The listing builds one solid part. Answer for the finished solid, in the listing's coordinates (mm). Coordinates: 2 decimals unless noted, no trailing zeros. Loops run counter-clockwise (first coordinate to the right, second up) from the corner with the lowest first, then second, coordinate; pieces in that order, holes last. Notation, with made-up numbers: (68, 28.25) - (94, 28.25) arc R29 cw to (94, 51.25) - close; hole circle Ø3 at (49, -26.5). An arc over 180 degrees is marked (long way). Return JSON: item names as keys, results as strings. Group by question number.
1. Section A-A (z = 0) is taken. Write down the section's boundary in (x, y).
2. Section D-D (y = 3.35) is taken. State how many separate pieces and enclosed holes the cut face has, and give its area (3 significant figures).
3. Each of these flat-tipped pins is pushed along its axis until it touches: P1, Ø2.5, axis at x = -40.66, z = 32.42, coming from the -Y side; P2, Ø1, axis at x = -24.5, y = 2.5, coming from the +Z side; P3, Ø1, axis at x = 4, y = 3, coming from the -Z side. Where does it stop, or does it pass through?
4. The mould has two halves that part along X. Classify faces 1 (the face through (-42.98, 2.03, -17.76)), 2 (the face through (13.836, 1.972, -23.766)): pulls with the +X half, pulls with the -X half, needs draft (parallel to the pull), parting line crosses it, or undercut.
5. Find the intervals of material crossed by line 1 along X through (y, z) = (3, -5); line 2 along X through (y, z) = (3.8, -22); line 3 along Z through (x, y) = (21, 1.3), in increasing order.
6. Section C-C (z = -36) is taken. Write down the section's boundary in (x, y).
7. Section B-B (x = 0) is taken. Write down the section's boundary in (y, z), and give its area (3 significant figures).
```python
from build123d import *

# Parameters (mm, degrees)
SKETCH_1_R      = 56
SKETCH_1_R_2    = 2.6
SKETCH_1_R_3    = 17.5
SKETCH_1_R_4    = 1.5
EXTRUDE_1_DEPTH = 4
FILLET_1_R      = 3


with BuildPart() as part:
    # 草图1 → 凸台-拉伸1 (new body)
    with BuildSketch(Plane(origin=(0, 0, 0), x_dir=(1, 0, 0), z_dir=(0, 1, 0))):
        with Locations(Location((0, 0, 0), (0, 0, 270))):
            Circle(SKETCH_1_R)
        with BuildLine():
            Line((-5, 47.236109069), (-5, 27.041634566))
            ThreePointArc((-5, 27.041634566), (-13.75, 23.815698604), (-20.918742494, 17.850944302))
            Line((-20.918742494, 17.850944302), (-38.40767043, 27.948181554))
            ThreePointArc((-38.40767043, 27.948181554), (-23.75, 41.13620668), (-5, 47.236109069))
        make_face(mode=Mode.SUBTRACT)
        with BuildLine():
            Line((-43.40767043, 19.287927516), (-25.918742494, 9.190690264))
            ThreePointArc((-25.918742494, 9.190690264), (-27.5, 0), (-25.918742494, -9.190690264))
            Line((-25.918742494, -9.190690264), (-43.40767043, -19.287927516))
            ThreePointArc((-43.40767043, -19.287927516), (-47.5, 0), (-43.40767043, 19.287927516))
        make_face(mode=Mode.SUBTRACT)
        with BuildLine():
            Line((-38.40767043, -27.948181554), (-20.918742494, -17.850944302))
            ThreePointArc((-20.918742494, -17.850944302), (-13.75, -23.815698604), (-5, -27.041634566))
            Line((-5, -27.041634566), (-5, -47.236109069))
            ThreePointArc((-5, -47.236109069), (-23.75, -41.13620668), (-38.40767043, -27.948181554))
        make_face(mode=Mode.SUBTRACT)
        with BuildLine():
            Line((5, -47.236109069), (5, -27.041634566))
            ThreePointArc((5, -27.041634566), (13.75, -23.815698604), (20.918742494, -17.850944302))
            Line((20.918742494, -17.850944302), (38.40767043, -27.948181554))
            ThreePointArc((38.40767043, -27.948181554), (23.75, -41.13620668), (5, -47.236109069))
        make_face(mode=Mode.SUBTRACT)
        with BuildLine():
            Line((43.40767043, -19.287927516), (25.918742494, -9.190690264))
            ThreePointArc((25.918742494, -9.190690264), (27.5, 0), (25.918742494, 9.190690264))
            Line((25.918742494, 9.190690264), (43.40767043, 19.287927516))
            ThreePointArc((43.40767043, 19.287927516), (47.5, 0), (43.40767043, -19.287927516))
        make_face(mode=Mode.SUBTRACT)
        with BuildLine():
            Line((38.40767043, 27.948181554), (20.918742494, 17.850944302))
            ThreePointArc((20.918742494, 17.850944302), (13.75, 23.815698604), (5, 27.041634566))
            Line((5, 27.041634566), (5, 47.236109069))
            ThreePointArc((5, 47.236109069), (23.75, 41.13620668), (38.40767043, 27.948181554))
        make_face(mode=Mode.SUBTRACT)
        with Locations(Location((0, 22.5, 0), (0, 0, 270))):
            Circle(SKETCH_1_R_2, mode=Mode.SUBTRACT)
        with Locations(Location((-19.485571585, -11.25, 0), (0, 0, 270))):
            Circle(SKETCH_1_R_2, mode=Mode.SUBTRACT)
        with Locations(Location((0, -22.5, 0), (0, 0, 270))):
            Circle(SKETCH_1_R_2, mode=Mode.SUBTRACT)
        with Locations(Location((19.485571585, -11.25, 0), (0, 0, 270))):
            Circle(SKETCH_1_R_2, mode=Mode.SUBTRACT)
        with Locations(Location((-19.485571585, 11.25, 0), (0, 0, 270))):
            Circle(SKETCH_1_R_2, mode=Mode.SUBTRACT)
        with Locations(Location((0, 0, 0), (0, 0, 270))):
            Circle(SKETCH_1_R_3, mode=Mode.SUBTRACT)
        with Locations(Location((19.485571585, 11.25, 0), (0, 0, 270))):
            Circle(SKETCH_1_R_2, mode=Mode.SUBTRACT)
        with Locations(Location((-32.421469697, -40.655237088, 0), (0, 0, 270))):
            Circle(SKETCH_1_R_4, mode=Mode.SUBTRACT)
        with Locations(Location((-40.655237088, -32.421469697, 0), (0, 0, 270))):
            Circle(SKETCH_1_R_4, mode=Mode.SUBTRACT)
        with Locations(Location((-22.561954434, -46.850381131, 0), (0, 0, 270))):
            Circle(SKETCH_1_R_4, mode=Mode.SUBTRACT)
        with Locations(Location((-11.571088566, -50.696251433, 0), (0, 0, 270))):
            Circle(SKETCH_1_R_4, mode=Mode.SUBTRACT)
        with Locations(Location((-46.850381131, -22.561954434, 0), (0, 0, 270))):
            Circle(SKETCH_1_R_4, mode=Mode.SUBTRACT)
        with Locations(Location((-50.696251433, -11.571088566, 0), (0, 0, 270))):
            Circle(SKETCH_1_R_4, mode=Mode.SUBTRACT)
        with Locations(Location((-52, 0, 0), (0, 0, 270))):
            Circle(SKETCH_1_R_4, mode=Mode.SUBTRACT)
        with Locations(Location((0, -52, 0), (0, 0, 270))):
            Circle(SKETCH_1_R_4, mode=Mode.SUBTRACT)
        with Locations(Location((11.571088566, -50.696251433, 0), (0, 0, 270))):
            Circle(SKETCH_1_R_4, mode=Mode.SUBTRACT)
        with Locations(Location((22.561954434, -46.850381131, 0), (0, 0, 270))):
            Circle(SKETCH_1_R_4, mode=Mode.SUBTRACT)
        with Locations(Location((32.421469697, -40.655237088, 0), (0, 0, 270))):
            Circle(SKETCH_1_R_4, mode=Mode.SUBTRACT)
        with Locations(Location((40.655237088, -32.421469697, 0), (0, 0, 270))):
            Circle(SKETCH_1_R_4, mode=Mode.SUBTRACT)
        with Locations(Location((46.850381131, -22.561954434, 0), (0, 0, 270))):
            Circle(SKETCH_1_R_4, mode=Mode.SUBTRACT)
        with Locations(Location((50.696251433, -11.571088566, 0), (0, 0, 270))):
            Circle(SKETCH_1_R_4, mode=Mode.SUBTRACT)
        with Locations(Location((-50.696251433, 11.571088566, 0), (0, 0, 270))):
            Circle(SKETCH_1_R_4, mode=Mode.SUBTRACT)
        with Locations(Location((-46.850381131, 22.561954434, 0), (0, 0, 270))):
            Circle(SKETCH_1_R_4, mode=Mode.SUBTRACT)
        with Locations(Location((-40.655237088, 32.421469697, 0), (0, 0, 270))):
            Circle(SKETCH_1_R_4, mode=Mode.SUBTRACT)
        with Locations(Location((-32.421469697, 40.655237088, 0), (0, 0, 270))):
            Circle(SKETCH_1_R_4, mode=Mode.SUBTRACT)
        with Locations(Location((-22.561954434, 46.850381131, 0), (0, 0, 270))):
            Circle(SKETCH_1_R_4, mode=Mode.SUBTRACT)
        with Locations(Location((-11.571088566, 50.696251433, 0), (0, 0, 270))):
            Circle(SKETCH_1_R_4, mode=Mode.SUBTRACT)
        with Locations(Location((40.655237088, 32.421469697, 0), (0, 0, 270))):
            Circle(SKETCH_1_R_4, mode=Mode.SUBTRACT)
        with Locations(Location((22.561954434, 46.850381131, 0), (0, 0, 270))):
            Circle(SKETCH_1_R_4, mode=Mode.SUBTRACT)
        with Locations(Location((11.571088566, 50.696251433, 0), (0, 0, 270))):
            Circle(SKETCH_1_R_4, mode=Mode.SUBTRACT)
        with Locations(Location((0, 52, 0), (0, 0, 270))):
            Circle(SKETCH_1_R_4, mode=Mode.SUBTRACT)
        with Locations(Location((46.850381131, 22.561954434, 0), (0, 0, 270))):
            Circle(SKETCH_1_R_4, mode=Mode.SUBTRACT)
        with Locations(Location((32.421469697, 40.655237088, 0), (0, 0, 270))):
            Circle(SKETCH_1_R_4, mode=Mode.SUBTRACT)
        with Locations(Location((52, 0, 0), (0, 0, 270))):
            Circle(SKETCH_1_R_4, mode=Mode.SUBTRACT)
        with Locations(Location((50.696251433, 11.571088566, 0), (0, 0, 270))):
            Circle(SKETCH_1_R_4, mode=Mode.SUBTRACT)
    extrude(amount=EXTRUDE_1_DEPTH)

    # 圆角1
    fillet_1_edges = [part.edges().sort_by_distance(p)[0] for p in [
        (5, 2, 27.041634566),
        (5, 2, 47.236109069),
        (38.40767043, 2, 27.948181554),
        (20.918742494, 2, 17.850944302),
        (43.40767043, 2, -19.287927516),
        (25.918742494, 2, -9.190690264),
        (25.918742494, 2, 9.190690264),
        (43.40767043, 2, 19.287927516),
        (5, 2, -47.236109069),
        (5, 2, -27.041634566),
        (20.918742494, 2, -17.850944302),
        (38.40767043, 2, -27.948181554),
        (-38.40767043, 2, -27.948181554),
        (-20.918742494, 2, -17.850944302),
        (-5, 2, -27.041634566),
        (-5, 2, -47.236109069),
        (-43.40767043, 2, 19.287927516),
        (-25.918742494, 2, 9.190690264),
        (-25.918742494, 2, -9.190690264),
        (-43.40767043, 2, -19.287927516),
        (-5, 2, 47.236109069),
        (-5, 2, 27.041634566),
        (-20.918742494, 2, 17.850944302),
        (-38.40767043, 2, 27.948181554),
    ]]
    fillet(fillet_1_edges, radius=FILLET_1_R)


solid = part.part
```
The answers:
{
 "1": {"outline": "(-56, 0) - (-53.5, 0) - (-53.5, 4) - (-56, 4) - close; (-50.5, 0) - (-47.5, 0) - (-47.5, 4) - (-50.5, 4) - close; (-27.5, 0) - (-17.5, 0) - (-17.5, 4) - (-27.5, 4) - close; (17.5, 0) - (27.5, 0) - (27.5, 4) - (17.5, 4) - close; (47.5, 0) - (50.5, 0) - (50.5, 4) - (47.5, 4) - close; (53.5, 0) - (56, 0) - (56, 4) - (53.5, 4) - close"},
 "2": {"separate pieces": "1", "enclosed holes": "41", "area": "5,100 mm2"},
 "3": {"P1": "passes through", "P2": "stops at z = 50.6", "P3": "stops at z = -55.89"},
 "4": {"face 1": "undercut", "face 2": "undercut"},
 "5": {"line 1": "x = -55.78 to -47.24, -27.04 to -16.77, 16.77 to 27.04, 47.24 to 55.78", "line 2": "x = -51.5 to -48.24, -45.46 to -28.11, -16.5 to -2.55, 2.55 to 16.5, 28.11 to 45.46, 48.24 to 51.5", "line 3": "z = -51.91 to -42.61, -18.68 to -13.36, -9.14 to 9.14, 13.36 to 18.68, 42.61 to 51.91"},
 "6": {"outline": "(-42.9, 0) - (-30.99, 0) - (-30.99, 4) - (-42.9, 4) - close; (-5, 0) - (5, 0) - (5, 4) - (-5, 4) - close; (30.99, 0) - (42.9, 0) - (42.9, 4) - (30.99, 4) - close"},
 "7": {"outline": "(0, -56) - (4, -56) - (4, -53.5) - (0, -53.5) - close; (0, -50.5) - (4, -50.5) - (4, -25.1) - (0, -25.1) - close; (0, -19.9) - (4, -19.9) - (4, -17.5) - (0, -17.5) - close; (0, 17.5) - (4, 17.5) - (4, 19.9) - (0, 19.9) - close; (0, 25.1) - (4, 25.1) - (4, 50.5) - (0, 50.5) - close; (0, 53.5) - (4, 53.5) - (4, 56) - (0, 56) - close", "area": "242 mm2"}
}
